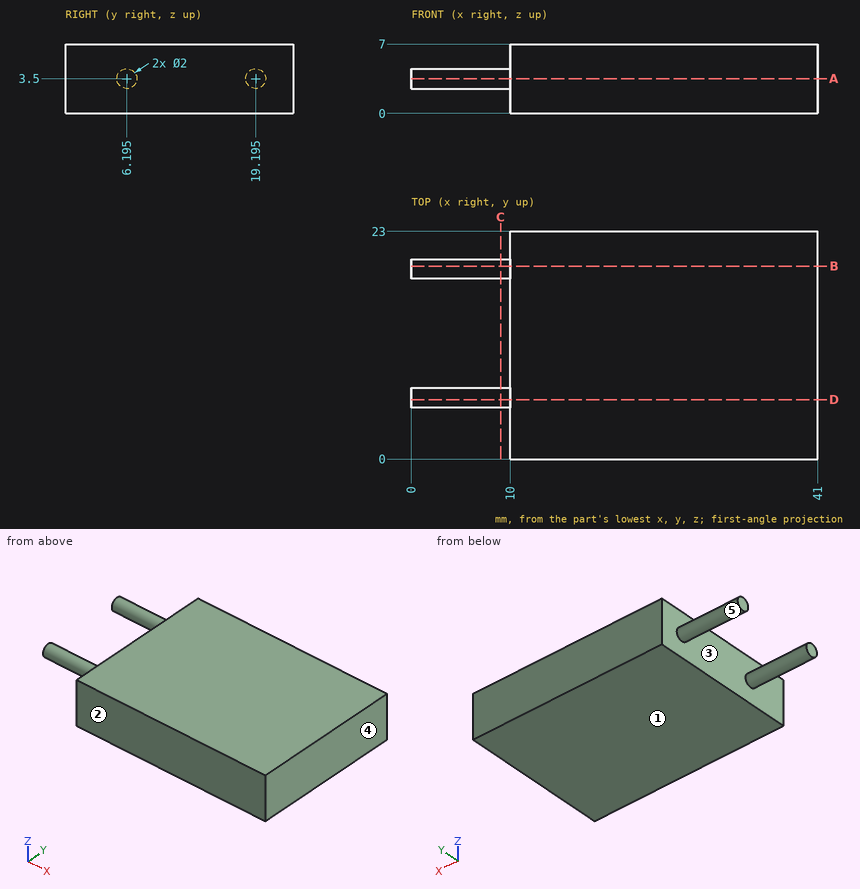
Answer from the drawing. Dimensions are ordinates in mm from the lowest x, y and z of the part. A direction names the side the tool comes from. Round coordinates to 2 decimals unless told otherwise and drop trailing zeros. Write each loop counter-clockwise with the first axis right and the second up, starting at its lowest first coordinate (ties: lowest second). Pieces come first, ordered by that corner, then holes. Notation, with made-up numbers: M 8,48.25 L 18,48.25 A23 cw 18,67.25 Z; hole C 34,89.5 d1. An arc over 180 degrees is marked long. Write each question's results on one line, items separated by ' | '. Start each with the question number.
Item 1: A cutting plane is placed at C-C on x = 9. Write down the section's boundary in (y, z) (1 decimal).
Item 2: A cutting plane is placed at D-D on y = 6. Write down the section's boundary in (x, z), and give its area (3 significant figures).
Item 3: A straight line is drawn through the part: L1, parallel to X at y = 14.5, z = 4.75. Find the intervals that lie inside material, in ascending order. Write a range as [from, to].
Item 4: For the marked faces 4 and 5, determine the directions among +Z, -Z, +X, -X, +Y, -Y from which every point of the face is accessible in a straight line to the end or side of a thin tool.
Item 5: Flat-ended cylindrical pins translate along their axes: pin 1 Ø3 at (x, z) = (6, 3.5) entering from -Y (3 decimals); pin 2 Ø3.5 at (y, z) = (14, 3.5) entering from -X; pin 3 Ø4 at (x, z) = (8.5, 5.5) entering from +Y. Find the tip coordinate at first contact, or state that the pin passes through.
Item 6: A cutting plane is placed at B-B on y = 19.5. Write down the section's boundary in (x, z), and give its area (3 significant figures).
Item 7: A cutting plane is placed at A-A on z = 3.5. Write down the section's boundary in (x, y) (1 decimal).
Item 8: For a pull along Y with two mould halves and no side action, classify the marked faces 1, 2 and 3 as pulls with the +Y half, pulls with the -Y half, needs draft (parallel to the pull), parting line crosses it, or undercut.
Check sheet entries:
1) outline: C 6.2,3.5 d2; C 19.2,3.5 d2
2) outline: M 0,2.52 L 10,2.52 L 10,0 L 41,0 L 41,7 L 10,7 L 10,4.48 L 0,4.48 Z | area: 237 mm²
3) L1: [10, 41]
4) face 4: +Z, -Z, +X, +Y, -Y | face 5: -X
5) pin 1: y = 5.195 | pin 2: x = 10 | pin 3: y = 23
6) outline: M 0,2.55 L 10,2.55 L 10,0 L 41,0 L 41,7 L 10,7 L 10,4.45 L 0,4.45 Z | area: 236 mm²
7) outline: M 0,5.2 L 10,5.2 L 10,0 L 41,0 L 41,23 L 10,23 L 10,20.2 L 0,20.2 L 0,18.2 L 10,18.2 L 10,7.2 L 0,7.2 Z
8) face 1: needs draft | face 2: pulls with the -Y half | face 3: undercut
